```python
from build123d import *

# Parameters (mm, degrees)
SKETCH1_R           = 35
BOSS_EXTRUDE1_DEPTH = 4
SKETCH2_R           = 42.5
SKETCH2_R_2         = 35
BOSS_EXTRUDE2_DEPTH = 48
SKETCH3_R           = 1.6
CUT_EXTRUDE1_DEPTH  = 48
SKETCH4_R           = 1.6
CUT_EXTRUDE2_DEPTH  = 10
SKETCH8_R           = 1.6
CUT_EXTRUDE6_DEPTH  = 15
SKETCH10_R          = 1.6
CUT_EXTRUDE8_DEPTH  = 10
BOSS_EXTRUDE3_DEPTH = 30.5
CHAMFER1_SIZE       = 20
CUT_EXTRUDE11_DEPTH = 21.5
SKETCH15_R          = 1.6
CUT_EXTRUDE13_DEPTH = 46
SKETCH16_W          = 9.455259108
SKETCH16_H          = 6.083224026
CUT_EXTRUDE15_DEPTH = 35


with BuildPart() as part:
    # Sketch1 → Boss-Extrude1 (new body)
    with BuildSketch(Plane(origin=(0, 0, 0), x_dir=(1, 0, 0), z_dir=(0, 1, 0))):
        with BuildLine():
            Line((62.449979984, -30), (150, -30))
            ThreePointArc((150, -30), (157.071067812, -27.071067812), (160, -20))
            Line((160, -20), (160, 20))
            ThreePointArc((160, 20), (157.071067812, 27.071067812), (150, 30))
            Line((150, 30), (62.449979984, 30))
            ThreePointArc((62.449979984, 30), (53.789725946, 31.972243623), (46.837484988, 37.5))
            ThreePointArc((46.837484988, 37.5), (-60, 0), (46.837484988, -37.5))
            ThreePointArc((46.837484988, -37.5), (53.789725946, -31.972243623), (62.449979984, -30))
        make_face()
        with Locations(Location((0, 0, 0), (0, 0, 270))):
            Circle(SKETCH1_R, mode=Mode.SUBTRACT)
    extrude(amount=BOSS_EXTRUDE1_DEPTH)

    # Sketch2 → Boss-Extrude2 (add)
    with BuildSketch(Plane(origin=(0, 4, 0), x_dir=(1, 0, 0), z_dir=(0, 1, 0))):
        with Locations(Location((0, 0, 0), (0, 0, 270))):
            Circle(SKETCH2_R)
        with Locations(Location((0, 0, 0), (0, 0, 270))):
            Circle(SKETCH2_R_2, mode=Mode.SUBTRACT)
    extrude(amount=BOSS_EXTRUDE2_DEPTH)

    # Sketch3 → Cut-Extrude1 (cut)
    with BuildSketch(Plane(origin=(0, 4, 0), x_dir=(1, 0, 0), z_dir=(0, 1, 0))):
        with Locations(Location((150, 20, 0), (0, 0, 270))):
            Circle(SKETCH3_R)
        with Locations(Location((150, -21.433629542, 0), (0, 0, 270))):
            Circle(SKETCH3_R)
        with BuildLine():
            ThreePointArc((-45.13862288, 27.337180296), (-51.248131898, -12.587520766), (-27.337180296, -45.13862288))
            ThreePointArc((-27.337180296, -45.13862288), (-24.590394929, -44.463959891), (-25.265057918, -41.717174524))
            ThreePointArc((-25.265057918, -41.717174524), (-47.363590779, -11.633403217), (-41.717174524, 25.265057918))
            ThreePointArc((-41.717174524, 25.265057918), (-42.391837513, 28.011843285), (-45.13862288, 27.337180296))
        make_face()
        with BuildLine():
            ThreePointArc((46.261369296, 26.251446503), (14.740318447, 51.504787048), (-25.405238706, 47.072846589))
            ThreePointArc((-25.405238706, 47.072846589), (-26.194356102, 44.356729189), (-23.478238701, 43.567611793))
            ThreePointArc((-23.478238701, 43.567611793), (13.624337923, 47.663616983), (42.756134499, 24.324446498))
            ThreePointArc((42.756134499, 24.324446498), (45.4722519, 23.535329102), (46.261369296, 26.251446503))
        make_face()
        with BuildLine():
            ThreePointArc((-0.378899838, -52.36040173), (37.251660029, -37.689041213), (53.48626558, -0.705998641))
            ThreePointArc((53.48626558, -0.705998641), (51.528597609, 1.335455771), (49.487143197, -0.6222122))
            ThreePointArc((49.487143197, -0.6222122), (34.483099434, -34.801988697), (-0.295113397, -48.361279348))
            ThreePointArc((-0.295113397, -48.361279348), (-2.336567809, -50.318947318), (-0.378899838, -52.36040173))
        make_face()
    extrude(amount=-CUT_EXTRUDE1_DEPTH, mode=Mode.SUBTRACT)

    # Sketch4 → Cut-Extrude2 (cut)
    with BuildSketch(Plane(origin=(0, 4, 0), x_dir=(1, 0, 0), z_dir=(0, 1, 0))):
        with Locations(Location((89.34, -8.89, 0), (0, 0, 270))):
            Circle(SKETCH4_R)
        with Locations(Location((89.34, 19.05, 0), (0, 0, 270))):
            Circle(SKETCH4_R)
        with Locations(Location((140.14, -24.13, 0), (0, 0, 270))):
            Circle(SKETCH4_R)
        with Locations(Location((141.41, 24.13, 0), (0, 0, 270))):
            Circle(SKETCH4_R)
    extrude(amount=-CUT_EXTRUDE2_DEPTH, mode=Mode.SUBTRACT)

    # Sketch8 → Cut-Extrude6 (cut)
    with BuildSketch(Plane(origin=(0, 52, 0), x_dir=(1, 0, 0), z_dir=(0, 1, 0))):
        with Locations(Location((-26.597013041, -28.18086935, 0), (0, 0, 270))):
            Circle(SKETCH8_R)
        with Locations(Location((-28.18086935, 26.597013041, 0), (0, 0, 270))):
            Circle(SKETCH8_R)
        with Locations(Location((26.597013041, 28.18086935, 0), (0, 0, 270))):
            Circle(SKETCH8_R)
        with Locations(Location((28.18086935, -26.597013041, 0), (0, 0, 270))):
            Circle(SKETCH8_R)
    extrude(amount=-CUT_EXTRUDE6_DEPTH, mode=Mode.SUBTRACT)

    # Sketch10 → Cut-Extrude8 (cut)
    with BuildSketch(Plane(origin=(0, 4, 0), x_dir=(1, 0, 0), z_dir=(0, 1, 0))):
        with Locations(Location((84.581, 26.035, 0), (0, 0, 270))):
            Circle(SKETCH10_R)
        with Locations(Location((114.426, 10.033, 0), (0, 0, 270))):
            Circle(SKETCH10_R)
    extrude(amount=-CUT_EXTRUDE8_DEPTH, mode=Mode.SUBTRACT)

    # Sketch12 → Boss-Extrude3 (add)
    with BuildSketch(Plane.XZ):
        with BuildLine():
            Line((-30.025, -10.060927898), (-30.025, 9.939072102))
            Line((-30.025, 9.939072102), (-33.559124627, 9.939072102))
            ThreePointArc((-33.559124627, 9.939072102), (-34.999942254, -0.063578173), (-33.522794183, -10.060927898))
            Line((-33.522794183, -10.060927898), (-30.025, -10.060927898))
        make_face()
        with BuildLine():
            Line((12.25, -10), (12.25, 10))
            Line((12.25, 10), (33.541019662, 10))
            ThreePointArc((33.541019662, 10), (35, 0), (33.541019662, -10))
            Line((33.541019662, -10), (12.25, -10))
        make_face()
    extrude(amount=-BOSS_EXTRUDE3_DEPTH)

    # Chamfer1
    chamfer1_edges = [part.edges().sort_by_distance(p)[0] for p in [
        (12.25, 0, 0),
    ]]
    chamfer(chamfer1_edges, length=CHAMFER1_SIZE)

    # Sketch14 → Cut-Extrude11 (cut)
    with BuildSketch(Plane(origin=(0, 52, 0), x_dir=(1, 0, 0), z_dir=(0, 1, 0))):
        with BuildLine():
            Line((0, 0), (-35.606142497, -18.226426322))
            ThreePointArc((-35.606142497, -18.226426322), (-40, 0), (-35.606142497, 18.226426322))
            Line((-35.606142497, 18.226426322), (0, 0))
        make_face()
    extrude(amount=-CUT_EXTRUDE11_DEPTH, mode=Mode.SUBTRACT)

    # Sketch15 → Cut-Extrude13 (cut)
    with BuildSketch(Plane(origin=(0, 52, 0), x_dir=(1, 0, 0), z_dir=(0, 1, 0))):
        with Locations(Location((-33.5, -5, 0), (0, 0, 270))):
            Circle(SKETCH15_R)
        with Locations(Location((-33.5, 5, 0), (0, 0, 270))):
            Circle(SKETCH15_R)
        with Locations(Location((15.1, -5, 0), (0, 0, 180))):
            Circle(SKETCH15_R)
        with Locations(Location((15.1, 5, 0), (0, 0, 180))):
            Circle(SKETCH15_R)
    extrude(amount=-CUT_EXTRUDE13_DEPTH, mode=Mode.SUBTRACT)

    # Sketch16 → Cut-Extrude15 (cut)
    with BuildSketch(Plane.ZY.offset(-12.25)):
        with Locations((0, 7)):
            Rectangle(SKETCH16_W, SKETCH16_H)
    extrude(amount=-CUT_EXTRUDE15_DEPTH, mode=Mode.SUBTRACT)


solid = part.part
```
Geometry check sheet. Reference: the model listing, model coordinates, mm. A direction names the side the tool comes from. Round coordinates to 2 decimals unless told otherwise and drop trailing zeros. Order: outer loops, then holes, each group sorted by start corner. A loop starts at its lowest first (then second) coordinate and runs counter-clockwise, first axis right, second up. Notation, with made-up numbers: (78, 55.5) - (104, 55.5) arc R5 cw to (104, 59.5) - close; hole circle Ø5 at (60, 31.25). An arc over 180 degrees is marked (long way). Use a Markdown table: item, result. Add a question column.
(1) Material ranges on line 1 along Z through (x, y) = (0, 36); line 2 along X through (y, z) = (43.5, 28.5); line 3 along Z through (x, y) = (29, 24.5), recorded low to high. Write a range as [from, to].
(2) Sectioned sample at B-B, the plane x = 75. Enter the section's corners in (y, z).
(3) Tool access check on faces 1 (the flat face through (107, 2, -30)), 2 (the flat face through (-33.41, 41.4, -17.1)), 3 (the cylindrical face through (-2.335, 2.028, 50.275)). Record the directions out of +Z, -Z, +X, -X, +Y, -Y that give a thin tool (end or side, any length) a straight path to the whole face; none if there is none.
(4) Release check for a two-part mould opening along X. For faces 4 (the cylindrical face through (-25.861, 27.664, -33.727)), 5 (the cylindrical face through (53.677, 1.972, 32.027)), 6 (the flat face through (48, 0, -1)), 7 (the cylindrical face through (15.3, 2.03, -51.34)) record: pulls with the +X half, pulls with the -X half, needs draft (parallel to the pull), parting line crosses it, or undercut.
(5) Sectioned sample at A-A, the plane y = 34. Enter the section's corners in (x, z), and give its area (3 significant figures).
(6) Depth check by flat-ended pin: pin 1 (3 mm diameter, centred on x = 111.5, y = 2, fed in from -Z); pin 2 (3 mm diameter, centred on x = -18.5, y = 12, fed in from +Z); pin 3 (5 mm diameter, centred on y = 24, z = -1, fed in from -X). Enter the tip coordinate at first touch or a pass-through.
Answers below:
| question | item | result |
|---|---|---|
| 1 | line 1 | [-42.5, -35], [35, 42.5] |
| 1 | line 2 | [-31.53, -28.16], [-25.03, -20.32], [20.32, 31.53] |
| 1 | line 3 | [-31.07, -19.6], [-10, 10], [19.6, 31.07] |
| 2 | outline | (0, -30) - (4, -30) - (4, 30) - (0, 30) - close |
| 3 | face 1 | -Z, +X, +Y, -Y |
| 3 | face 2 | +Y |
| 3 | face 3 | +Y, -Y |
| 4 | face 4 | parting line crosses it |
| 4 | face 5 | pulls with the +X half |
| 4 | face 6 | needs draft |
| 4 | face 7 | undercut |
| 5 | outline | circle Ø85 at (0, 0); hole (-35.61, -18.23) - (-31.16, -15.95) arc R35 ccw (long way) to (-31.16, 15.95) - (-35.61, 18.23) arc R40 ccw to start |
| 5 | area | 1,650 mm² |
| 6 | pin 1 | z = -30 |
| 6 | pin 2 | z = 38.95 |
| 6 | pin 3 | x = -42.5 |
